Autodesk Fusion 360 part; units mm, degrees
sketch "Sketch1" plane through (0, 0, 0) normal (0, 0, 1) x (1, 0, 0)
  circle A0 centre (0, 0) radius 19
  dimension "d1" = 38
extrude "Extrude1" add sketch "Sketch1" along normal blind 35
sketch "Sketch2" plane through (0, 0, 35) normal (0, 0, 1) x (-1, 0, 0)
  circle A0 centre (0, 0) radius 19
  circle A1 centre (0, 0) radius 10
  circle A2 centre (0, 0) radius 14 construction
  circle A3 centre (0, 0) radius 15 construction
  circle A4 centre (0, 14) radius 1.55
  line L0 (0, 0) -> (0, 1) construction
  line L1 (0, 1) -> (0, 14) construction
  line L2 (0, 0) -> (-8.8168, 12.1353) construction
  circle A5 centre (-8.8168, 12.1353) radius 1.55
  circle A6 centre (-12.1244, -7) radius 1.55
  circle A7 centre (12.1244, -7) radius 1.55
  circle A8 centre (-6.101, -13.7032) radius 1.55
  circle A9 centre (14.9178, 1.5679) radius 1.55
  dimension "d4" = 20
  dimension "d13" = 28
  dimension "d14" = 30
  dimension "d15" = 3.1
  dimension "d16" = 36
  dimension "d17" = 3.1
  dimension "d19" = 360
  dimension "d21" = 360
extrude "Extrude2" add sketch "Sketch2" along normal blind 5 contours A1
sketch "Sketch3" plane through (0, 0, 40) normal (0, 0, 1) x (-1, 0, 0)
  circle A0 centre (0, 0) radius 10
  circle A1 centre (0, 0) radius 3
  line L0 (0, 3) -> (0, -2.58) construction
  line L1 (0, -2.58) -> (-1.5309, -2.58)
  line L2 (0, -2.58) -> (1.5309, -2.58)
  dimension "d7" = 6
  dimension "d8" = 5.58
extrude "Extrude3" add sketch "Sketch3" along normal blind 13 contours A1 L1 L2 picked at (0.0089, 1.1344)
extrude "Extrude4" add sketch "Sketch3" along normal blind 3 contours A1 L1 L2 picked at (0.1335, -2.8511)
extrude "Extrude5" cut sketch "Sketch2" against normal blind 6 contours A4 | A5 | A6 | A7 | A8 | A9
extrude "Extruir6" cut 1 faces at (-0.6852, 0.4836, 53) along direction (0, 0, -1) blind 10
extrude "Extruir7" cut 1 faces at (-0.782, -0.3761, 43) along direction (0, 0, -1) blind 5
extrude "Extruir8" add 1 faces at (-0.782, -0.3761, 38) along direction (0, 0, 1) blind 15
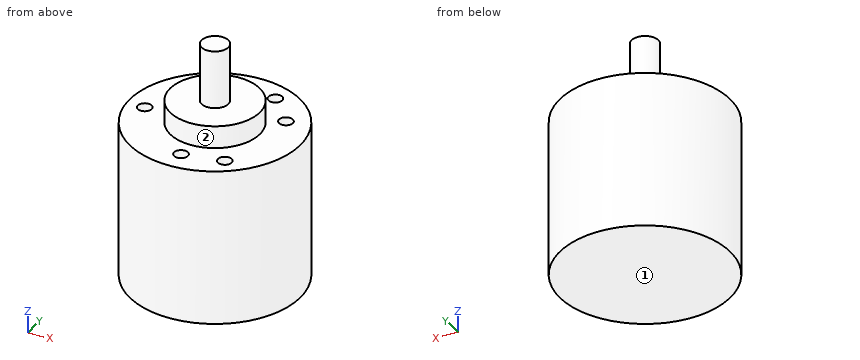
Work out the finished part from the listing and answer in its coordinate system (mm). Face numbers are marked on the shaded views. A direction names the side the tool comes from. Coordinates: 2 decimals unless noted, no trailing zeros. Loops run counter-clockwise (first coordinate to the right, second up) from the corner with the lowest first, then second, coordinate; pieces in that order, holes last. Notation, with made-up numbers: (70.5, 64) - (76.5, 64) arc R24 ccw to (76.5, 75) - close; hole circle Ø10 at (-4, -17.75). An arc over 180 degrees is marked (long way). Use a Markdown table: item, result.
Item 1: Given pin 1 Ø0.9 at (x, y) = (7, 13) entering from +Z; pin 2 Ø2.5 at (x, y) = (0, -14) entering from +Z; pin 3 Ø10 at (x, z) = (2, 31.5) entering from +Y, each flat-ended and moving along its own axis, determine where each tip first touches the part or whether it passes through.
Evaluation:
| item | result |
|---|---|
| pin 1 | stops at z = 35 |
| pin 2 | stops at z = 29 |
| pin 3 | stops at y = 19 |
Item 2: For the marked faces 1 and 2, determine the directions among +Z, -Z, +X, -X, +Y, -Y from which every point of the face is accessible in a straight line to the end or side of a thin tool.
Evaluation:
| item | result |
|---|---|
| face 1 | -Z, +X, -X, +Y, -Y |
| face 2 | +Z |
Item 3: Find section A-A, the plane x = 0. Determine the outline of the cut face in (y, z), and give its area (3 significant figures).
Evaluation:
| item | result |
|---|---|
| outline | (-19, 0) - (19, 0) - (19, 35) - (10, 35) - (10, 40) - (3, 40) - (3, 53) - (-3, 53) - (-3, 40) - (-10, 40) - (-10, 35) - (-12.45, 35) - (-12.45, 29) - (-15.55, 29) - (-15.55, 35) - (-19, 35) - close |
| area | 1,490 mm2 |
Item 4: Find section C-C, the plane z = 12. Determine the outline of the cut face in (x, y).
Evaluation:
| item | result |
|---|---|
| outline | circle Ø38 at (0, 0) |
Item 5: Consider probe 1 along X at (y, z) = (7, 31.1); probe 2 along Z at (x, y) = (-9.5, -8); probe 3 along Z at (x, y) = (-3, -5.5). Determine where each line is inside the solid, lowest interval first. Write a range as from..to.
Evaluation:
| item | result |
|---|---|
| probe 1 | x = -17.66..-13.67, -10.57..10.57, 13.67..17.66 |
| probe 2 | z = 0..35 |
| probe 3 | z = 0..40 |
Item 6: Find section D-D, the plane x = -12.5. Determine the outline of the cut face in (y, z), and give its area (3 significant figures).
Evaluation:
| item | result |
|---|---|
| outline | (-14.31, 0) - (14.31, 0) - (14.31, 35) - (8.5, 35) - (8.5, 29) - (5.5, 29) - (5.5, 35) - (-14.31, 35) - close |
| area | 984 mm2 |
Item 7: Find section B-B, the plane y = 7. Determine the outline of the cut face in (x, z).
Evaluation:
| item | result |
|---|---|
| outline | (-17.66, 0) - (17.66, 0) - (17.66, 35) - (13.67, 35) - (13.67, 29) - (10.57, 29) - (10.57, 35) - (7.14, 35) - (7.14, 40) - (-7.14, 40) - (-7.14, 35) - (-10.57, 35) - (-10.57, 29) - (-13.67, 29) - (-13.67, 35) - (-17.66, 35) - close |
